Check sheet for the modelled part. Datum: model origin and axes. Units: mm. Face numbers are marked on the shaded views. A direction names the side the tool comes from. Coordinates: 2 decimals unless noted, no trailing zeros. Loops run counter-clockwise (first coordinate to the right, second up) from the corner with the lowest first, then second, coordinate; pieces in that order, holes last.
Autodesk Inventor part; units mm, degrees
ref_plane "Work Plane1" through (-42.5, 0, -23.8855) normal (-1, 0, 0) x (0, -1, 0)
ref_plane "YZ Plane" through (0, 0, 0) normal (1, 0, 0) x (0, 1, 0)
ref_plane "XZ Plane" through (0, 0, 0) normal (0, 1, 0) x (-1, 0, 0)
sketch "Sketch1" plane through (0, 0, 0) normal (0, 1, 0) x (-1, 0, 0)
  line L0 (42.5, 0) -> (-42.5, 0) construction
  line L1 (42.5, 23.8855) -> (-42.5, 23.8855)
  line L2 (-42.5, -23.8855) -> (42.5, -23.8855)
  arc A0 (42.5, -23.8855) -> (42.5, 23.8855) centre (42.5, 0) ccw
  arc A1 (-42.5, 23.8855) -> (-42.5, -23.8855) centre (-42.5, 0) ccw
  point P0 (0, 0)
  point P1 (0, 0)
  dimension "d0" = 85
  dimension "d1" = 47.771
ref_plane "Work Plane1" through (-42.5, 0, -23.8855) normal (-1, 0, 0) x (0, -1, 0)
sketch "Sketch2" plane through (-42.5, 0, -23.8855) normal (-1, 0, 0) x (0, -1, 0)
  line L0 (7.5, 0) -> (-7.5, 0)
  line L1 (-7.5, 0) -> (-7.5, -1.2)
  line L2 (-7.5, -1.2) -> (7.5, -1.2)
  line L3 (7.5, -1.2) -> (7.5, 0)
  line L4 (7.5, 0) -> (-7.5, -1.2) construction
  line L5 (-7.5, 0) -> (7.5, -1.2) construction
  point P0 (0, 23.8855)
  point P1 (0, -0.6)
  point P2 (0, 0)
  dimension "d2" = 15
  dimension "d3" = 1.2
sweep "Sweep1" add profiles "Sketch2" path "Sketch1"
properties part number "2309HCMUTE-CDT23-BELT_S5M-320X64X15" material "Rubber"
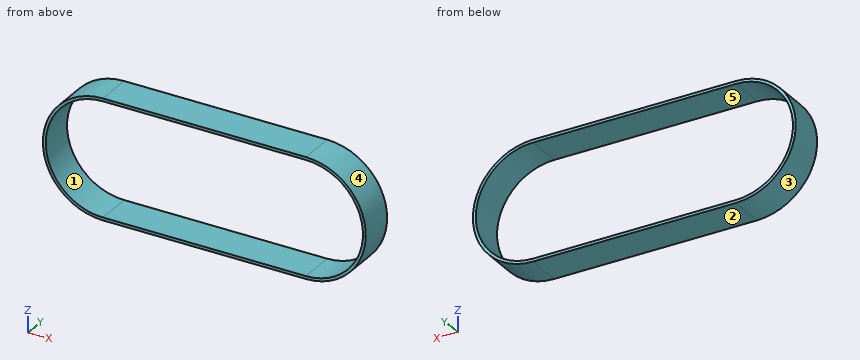
1) Scan lines: line 1 (Z direction, x = -25, y = -1.25); line 2 (X direction, y = -5, z = 5.5); line 3 (X direction, y = 4.75, z = -21). Record each from-to range of solid material in increasing order.
Answer sheet:
line 1: z = -25.09 to -23.89, 23.89 to 25.09
line 2: x = -66.98 to -65.74, 65.74 to 66.98
line 3: x = -56.22 to -53.88, 53.88 to 56.22
2) Set-up check for the marked faces 4 and 5: record each of +Z, -Z, +X, -X, +Y, -Y from which the full face is reachable in a straight line by a thin tool's end or side.
Answer sheet:
face 4: +X, +Y, -Y
face 5: +Y, -Y
3) Section check B-B on x = -32.5. Enter the section's corners in (y, z), plus the area to 3 significant figures.
Answer sheet:
outline: (-7.5, -25.09) - (7.5, -25.09) - (7.5, -23.89) - (-7.5, -23.89) - close; (-7.5, 23.89) - (7.5, 23.89) - (7.5, 25.09) - (-7.5, 25.09) - close
area: 36.0 mm2
4) Mould release check, pull along X, two halves, no side actions. Record for the marked faces 1, 2 and 3: +X half, -X half, draft (parallel to the pull), parting line (faces both ways), or undercut.
Answer sheet:
face 1: undercut
face 2: draft
face 3: -X half
5) Section check A-A on z = 0. Enter the section's corners in (x, y).
Answer sheet:
outline: (-67.59, -7.5) - (-66.39, -7.5) - (-66.39, 7.5) - (-67.59, 7.5) - close; (66.39, -7.5) - (67.59, -7.5) - (67.59, 7.5) - (66.39, 7.5) - close
6) Section check C-C on y = 6.25. Enter the section's corners in (x, z).
Answer sheet:
outline: (-42.5, -25.09) - (42.5, -25.09) arc R25.09 ccw to (42.5, 25.09) - (-42.5, 25.09) arc R25.09 ccw to start; hole (-42.5, -23.89) - (42.5, -23.89) arc R23.89 ccw to (42.5, 23.89) - (-42.5, 23.89) arc R23.89 ccw to start
7) Depth check by flat-ended pin: pin 1 (8 mm diameter, centred on y = 0.5, z = 2, fed in from +X); pin 2 (5 mm diameter, centred on y = 4, z = -14, fed in from -X). Enter the tip coordinate at first touch or a pass-through.
Answer sheet:
pin 1: stops at x = 67.59
pin 2: stops at x = -64.79
